Source: CAD feature listing. Evaluate the final solid. Frame: model axes, mm. Face numbers are marked on the shaded views. A direction names the side the tool comes from. Round coordinates to 2 decimals unless told otherwise and drop trailing zeros. Loops run counter-clockwise (first coordinate to the right, second up) from the corner with the lowest first, then second, coordinate; pieces in that order, holes last.
Item 1: Section query D-D on y = -17. Return loops of the section in (x, z).
Item 2: First-contact query: P1, Ø15, axis at x = -11.5, y = -25, coming from the +Z side; P2, Ø6, axis at x = -2, z = 16.5, coming from the -Y side. Flat tips, straight axial feed; report the tip coordinate or a pass-through.
Item 3: Section query C-C on x = 11.5. Return loops of the section in (y, z).
Item 4: Ray query, L1, parallel to Y at x = 0, z = 5.75; L2, parallel to Z at x = -17, y = -31; L3, parallel to Y at x = -15.5, z = 28. Return the intervals inside material, ascending.
Item 5: Section query A-A on x = 0. Return loops of the section in (y, z).
Item 6: Access query for the marked faces 1, 2 and 3. Directions: +Z, -Z, +X, -X, +Y, -Y. A direction counts if a zero-diameter tool reaches every point of the face in a straight line with its end or side. Return the directions, or none.
Item 7: Pull-direction query (Y, two-part tool) for the marked faces 4, 5 and 6; classes: released by +Y, released by -Y, zero draft, split by the parting line, or undercut.
Item 8: Section query B-B on y = -25. Return loops of the section in (x, z), then the cut area to 3 significant figures.
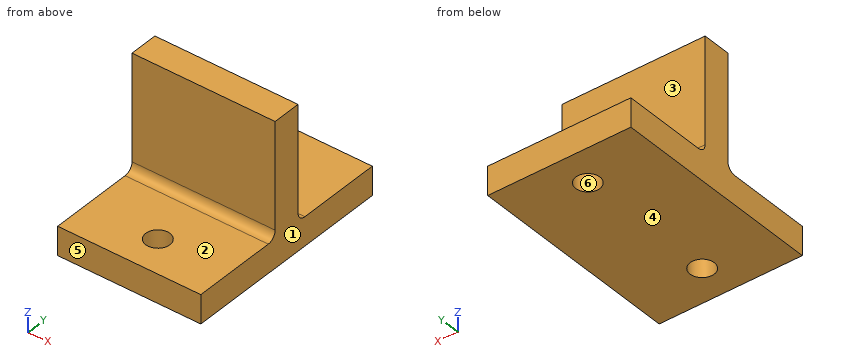
```python
from build123d import *

# Parameters (mm, degrees)
CROQUIS1_W                     = 50
CROQUIS1_H                     = 75
SALIENTE_EXTRUIR1_DEPTH        = 10
CROQUIS2_W                     = 50
CROQUIS2_H                     = 10
SALIENTE_EXTRUIR2_DEPTH        = 40
REDONDEO1_R                    = 3
TALADRO_DE_MARGEN_PARA_5_161_D = 8.4328


with BuildPart() as part:
    # Croquis1 → Saliente-Extruir1 (new body)
    with BuildSketch(Plane.XY):
        Rectangle(CROQUIS1_W, CROQUIS1_H)
    extrude(amount=SALIENTE_EXTRUIR1_DEPTH)

    # Croquis2 → Saliente-Extruir2 (add)
    with BuildSketch(Plane.XY.offset(10)):
        Rectangle(CROQUIS2_W, CROQUIS2_H)
    extrude(amount=SALIENTE_EXTRUIR2_DEPTH)

    # Redondeo1
    redondeo1_edges = [part.edges().sort_by_distance(p)[0] for p in [
        (0, -5, 10),
        (0, 5, 10),
    ]]
    fillet(redondeo1_edges, radius=REDONDEO1_R)

    # Taladro de margen para 5/161 (through all)
    with Locations(Plane(origin=(0, 25, 0), x_dir=(-1, 0, 0), z_dir=(0, 0, -1))):
        with Locations((0, 0), (0, -50)):
            Hole(TALADRO_DE_MARGEN_PARA_5_161_D / 2)


solid = part.part
```
Data:
1. outline: (-25, 0) - (25, 0) - (25, 10) - (-25, 10) - close
2. P1: stops at z = 10
2. P2: stops at y = -5
3. outline: (-37.5, 0) - (37.5, 0) - (37.5, 10) - (8, 10) arc R3 cw to (5, 13) - (5, 50) - (-5, 50) - (-5, 13) arc R3 cw to (-8, 10) - (-37.5, 10) - close
4. L1: y = -37.5 to -29.22, -20.78 to 20.78, 29.22 to 37.5
4. L2: z = 0 to 10
4. L3: y = -5 to 5
5. outline: (-37.5, 0) - (-29.22, 0) - (-29.22, 10) - (-37.5, 10) - close; (-20.78, 0) - (20.78, 0) - (20.78, 10) - (8, 10) arc R3 cw to (5, 13) - (5, 50) - (-5, 50) - (-5, 13) arc R3 cw to (-8, 10) - (-20.78, 10) - close; (29.22, 0) - (37.5, 0) - (37.5, 10) - (29.22, 10) - close
6. face 1: +Z, -Z, +X, +Y, -Y
6. face 2: +Z, +X, -X, -Y
6. face 3: +Z, +X, -X, +Y
7. face 4: zero draft
7. face 5: released by -Y
7. face 6: undercut
8. outline: (-25, 0) - (-4.22, 0) - (-4.22, 10) - (-25, 10) - close; (4.22, 0) - (25, 0) - (25, 10) - (4.22, 10) - close
8. area: 416 mm2
